Geometry: final body of the model. Coordinates: model frame, mm. Face numbers are marked on the shaded views. Round coordinates to 2 decimals unless told otherwise and drop trailing zeros. Loops run counter-clockwise (first coordinate to the right, second up) from the corner with the lowest first, then second, coordinate; pieces in that order, holes last. Notation, with made-up numbers: M 11.5,-27.75 L 67.5,-27.75 A16 cw 67.5,-21.75 Z; hole C -1,71.5 d5. An arc over 180 degrees is marked long. Answer as a JSON object with one key per item and string values.
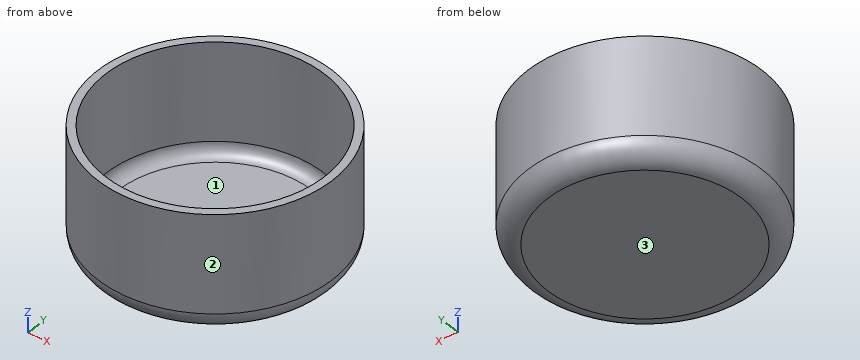
```python
from build123d import *

# Parameters (mm, degrees)
F2_T = -2.54


with BuildPart() as f1:
    # F0 (on Front) → F1 (revolve)
    with BuildSketch(Plane.XZ):
        with BuildLine():
            Line((0, 38.1), (0, 0))
            Line((0, 0), (31.75, 0))
            ThreePointArc((31.75, 0), (36.240128, 1.859872), (38.1, 6.35))
            Line((38.1, 6.35), (38.1, 38.1))
            Line((38.1, 38.1), (0, 38.1))
        make_face()
    revolve(axis=Axis((0, 0, 22.184535), (0, 0, 1)))

    # F2
    f2_openings = [f1.faces().sort_by_distance(p)[0] for p in [
        (0, 0, 38.1),
    ]]
    offset(amount=F2_T, openings=f2_openings)


solid = f1.part
```
1) Cut plane C-C on z = 10.5. Return the cut outline in (x, y), and give its area (3 significant figures).
Geometry results:
{"outline": "C 0,0 d76.2; hole C 0,0 d71.12", "area": "588 mm2"}
2) Cut plane D-D on z = 4. Return the cut outline in (x, y), and give its area (3 significant figures).
Geometry results:
{"outline": "C 0,0 d75.3; hole C 0,0 d69.5", "area": "660 mm2"}
3) Pull-direction query (X, two-part tool) for the marked faces 1, 2 and 3; classes: +X half, -X half, draft (parallel to the pull), parting line (faces both ways), or undercut.
Geometry results:
{"face 1": "undercut", "face 2": "parting line", "face 3": "draft"}
4) First-contact query: pin 1 (10 mm diameter, centred on x = 25, z = 31.5, fed in from -Y); pin 2 (19 mm diameter, centred on x = 2, y = 6, fed in from +Z); pin 3 (1 mm diameter, centred on y = -23, z = 16.5, fed in from -X). Flat tips, straight axial feed; report the tip coordinate or a pass-through.
Geometry results:
{"pin 1": "y = -32.43", "pin 2": "z = 2.54", "pin 3": "x = -30.75"}
5) Line query: probe 1 along Y at (x, z) = (0, 26); probe 2 along Z at (x, y) = (-12, 0). Output: solid intervals per line, ascending.
Geometry results:
{"probe 1": "-38.1 to -35.56, 35.56 to 38.1", "probe 2": "0 to 2.54"}
6) Cut plane A-A on y = 0. Return the cut outline in (x, z).
Geometry results:
{"outline": "M -38.1,6.35 A6.35 ccw -31.75,0 L 31.75,0 A6.35 ccw 38.1,6.35 L 38.1,38.1 L 35.56,38.1 L 35.56,6.35 A3.81 cw 31.75,2.54 L -31.75,2.54 A3.81 cw -35.56,6.35 L -35.56,38.1 L -38.1,38.1 Z"}
